Geometry: final body of the model. Coordinates: model frame, mm. A direction names the side the tool comes from. Give positions to 0.01 mm unless a question says otherwise; leave off trailing zeros. Order: outer loops, then holes, each group sorted by start corner. A loop starts at its lowest first (then second) coordinate and runs counter-clockwise, first axis right, second up. Notation, with made-up numbers: (0.25, 59) - (58.25, 59) arc R22 ccw to (58.25, 86) - close; hole circle Ø7 at (-33.75, 69). An arc over 180 degrees is marked (long way). Put each result on its own line as item: value. Start each with the question number.
1. Set-up query: faces 1 (the flat face through (4.1, 8, -9.6)), 2 (the flat face through (7.9, 8, -6.9)), 3 (the cylindrical face through (9.7, 2.96, -6.18)). Return all of +Z, -Z, +X, -X, +Y, -Y with unobstructed straight access to the full face (end or side cutting, diameter ignored); none if empty.
2. Section B-B on y = 9.5. Return the cut outline in (x, z).
3. Section C-C on z = 0. Return the cut outline in (x, y).
4. Section D-D on y = 2.5. Return the cut outline in (x, z), plus the area to 3 significant figures.
5. Section A-A on x = 0. Return the cut outline in (y, z), plus the area to 3 significant figures.
6. Ray query, line 1 along X through (y, z) = (2.75, 0); line 2 along Y through (x, z) = (-1.5, -2); line 3 along Y through (x, z) = (0, 4.75). Return the intervals inside material, ascending. Write a range as from..to.
7. First-contact query: P1, Ø5, axis at x = 0, z = 0, coming from the -Y side; P2, Ø8, axis at y = 2.5, z = -6, coming from the +X side; P3, Ø1.9, axis at y = 14.5, z = 0.5, coming from the +X side. Flat tips, straight axial feed; report the tip coordinate or a pass-through.
8. Mould query, pull axis Z, two halves, no side actions, for faces 4 (the cylindrical face through (-12.447, 2.465, 2.764)), 5 (the flat face through (0, 23.6, 0)), 6 (the flat face through (0, 11, 0)). Classes: pulls with the +Z half, pulls with the -Z half, needs draft (parallel to the pull), parting line crosses it, or undercut.
from build123d import *

# Parameters (mm, degrees)
SKETCH_1_R          = 14
EXTRUDE_1_DEPTH     = 10
SKETCH_2_R          = 11.5
CUT_EXTRUDE_1_DEPTH = 6
SKETCH_3_R          = 14
SKETCH_3_R_2        = 12.75
CUT_EXTRUDE_2_DEPTH = 5
CUT_EXTRUDE_START   = -4
CUT_EXTRUDE_3_DEPTH = 4
CHAMFER_1_SIZE      = 2
EXTRUDE_2_DEPTH     = 6.8
SKETCH_6_R          = 2.9
EXTRUDE_3_DEPTH     = 6.8
SKETCH_7_R          = 1.5
CUT_EXTRUDE_4_DEPTH = 5


with BuildPart() as part:
    # 草图1 → 凸台-拉伸1 (new body)
    with BuildSketch(Plane(origin=(0, 0, 0), x_dir=(1, 0, 0), z_dir=(0, 1, 0))):
        with Locations(Location((0, 0, 0), (0, 0, 270))):
            Circle(SKETCH_1_R)
    extrude(amount=EXTRUDE_1_DEPTH)

    # 草图2 → 切除-拉伸1 (cut)
    with BuildSketch(Plane.XZ):
        with Locations(Location((0, 0, 0), (0, 0, 270))):
            Circle(SKETCH_2_R)
    extrude(amount=-CUT_EXTRUDE_1_DEPTH, mode=Mode.SUBTRACT)

    # 草图3 → 切除-拉伸2 (cut)
    with BuildSketch(Plane.XZ):
        with Locations(Location((0, 0, 0), (0, 0, 270))):
            Circle(SKETCH_3_R)
        with Locations(Location((0, 0, 0), (0, 0, 270))):
            Circle(SKETCH_3_R_2, mode=Mode.SUBTRACT)
    extrude(amount=-CUT_EXTRUDE_2_DEPTH, mode=Mode.SUBTRACT)

    # 草图4 → 切除-拉伸3 (cut)
    with BuildSketch(Plane(origin=(0, 10, 0), x_dir=(1, 0, 0), z_dir=(0, 1, 0)).offset(CUT_EXTRUDE_START)):
        with BuildLine():
            Line((-5.46333165, 12.889996403), (-2.771638598, 6.39167453))
            ThreePointArc((-2.771638598, 6.39167453), (0, 4.539724827), (2.771638598, 6.39167453))
            Line((2.771638598, 6.39167453), (5.46333165, 12.889996403))
            ThreePointArc((5.46333165, 12.889996403), (0, 14), (-5.46333165, 12.889996403))
        make_face()
        with BuildLine():
            Line((-5.222360283, 4.611121001), (-10.570852749, 9.179165113))
            ThreePointArc((-10.570852749, 9.179165113), (-13.114723376, 4.899390856), (-14, 0))
            ThreePointArc((-14, 0), (-13.986838163, -0.6069252), (-13.9473774, -1.212709221))
            Line((-13.9473774, -1.212709221), (-6.935327141, -0.660848897))
            ThreePointArc((-6.935327141, -0.660848897), (-4.317534879, 1.402852121), (-5.222360283, 4.611121001))
        make_face()
        with BuildLine():
            Line((-5.999234754, -3.541845025), (-11.996477939, -7.216960375))
            ThreePointArc((-11.996477939, -7.216960375), (-8.228993532, -11.326237921), (-3.156621637, -13.63949192))
            Line((-3.156621637, -13.63949192), (-1.514629298, -6.800101609))
            ThreePointArc((-1.514629298, -6.800101609), (-2.668383303, -3.672714535), (-5.999234754, -3.541845025))
        make_face()
        with BuildLine():
            ThreePointArc((3.156621637, -13.63949192), (8.228993532, -11.326237921), (11.996477939, -7.216960375))
            Line((11.996477939, -7.216960375), (5.999234754, -3.541845025))
            ThreePointArc((5.999234754, -3.541845025), (2.668383303, -3.672714535), (1.514629298, -6.800101609))
            Line((1.514629298, -6.800101609), (3.156621637, -13.63949192))
        make_face()
        with BuildLine():
            ThreePointArc((14, 0), (13.114723376, 4.899390856), (10.570852749, 9.179165113))
            Line((10.570852749, 9.179165113), (5.222360283, 4.611121001))
            ThreePointArc((5.222360283, 4.611121001), (4.317534879, 1.402852121), (6.935327141, -0.660848897))
            Line((6.935327141, -0.660848897), (13.9473774, -1.212709221))
            ThreePointArc((13.9473774, -1.212709221), (13.986838163, -0.6069252), (14, 0))
        make_face()
    extrude(amount=CUT_EXTRUDE_3_DEPTH, mode=Mode.SUBTRACT)

    # 倒角1
    chamfer_1_edges = [part.edges().sort_by_distance(p)[0] for p in [
        (-8.228993532, 10, -11.326237921),
        (-13.314791228, 10, 4.326237921),
        (1.588570602, 10, 13.909580994),
        (13.314791228, 10, 4.326237921),
        (8.228993532, 10, -11.326237921),
    ]]
    chamfer(chamfer_1_edges, length=CHAMFER_1_SIZE)

    # 草图5 → 凸台-拉伸2 (add)
    with BuildSketch(Plane(origin=(0, 10, 0), x_dir=(1, 0, 0), z_dir=(0, 1, 0))):
        with BuildLine():
            Line((-3.45, 1.923538406), (-3.45, -1.923538406))
            ThreePointArc((-3.45, -1.923538406), (0, -3.95), (3.45, -1.923538406))
            Line((3.45, -1.923538406), (3.45, 1.923538406))
            ThreePointArc((3.45, 1.923538406), (0, 3.95), (-3.45, 1.923538406))
        make_face()
    extrude(amount=EXTRUDE_2_DEPTH)

    # 草图6 → 凸台-拉伸3 (add)
    with BuildSketch(Plane(origin=(0, 16.8, 0), x_dir=(1, 0, 0), z_dir=(0, 1, 0))):
        with Locations(Location((0, 0, 0), (0, 0, 270))):
            Circle(SKETCH_6_R)
    extrude(amount=EXTRUDE_3_DEPTH)

    # 草图7 → 切除-拉伸4 (cut)
    with BuildSketch(Plane.XZ.offset(-6)):
        with Locations(Location((0, 0, 0), (0, 0, 270))):
            Circle(SKETCH_7_R)
    extrude(amount=-CUT_EXTRUDE_4_DEPTH, mode=Mode.SUBTRACT)


solid = part.part
Resolved:
1. face 1: -Z, +Y
1. face 2: +X, +Y
1. face 3: -Y
2. outline: (-12.45, 1.1) - (-6.94, 0.66) arc R3 cw to (-5.22, -4.61) - (-9.43, -8.2) arc R12.5 ccw to (-4.89, -11.5) - (-2.77, -6.39) arc R3 cw to (2.77, -6.39) - (4.89, -11.5) arc R12.5 ccw to (9.43, -8.2) - (5.22, -4.61) arc R3 cw to (6.94, 0.66) - (12.45, 1.1) arc R12.5 ccw to (10.72, 6.43) - (6, 3.54) arc R3 cw to (1.51, 6.8) - (2.81, 12.18) arc R12.5 ccw to (-2.81, 12.18) - (-1.51, 6.8) arc R3 cw to (-6, 3.54) - (-10.72, 6.43) arc R12.5 ccw to start; hole circle Ø3 at (0, 0)
3. outline: (-14, 5) - (-12.75, 5) - (-12.75, 0) - (-11.5, 0) - (-11.5, 6) - (-14, 6) - close; (-5.28, 6) - (-1.5, 6) - (-1.5, 11) - (1.5, 11) - (1.5, 6) - (5.28, 6) - (5.28, 10) - (3.45, 10) - (3.45, 16.8) - (2.9, 16.8) - (2.9, 23.6) - (-2.9, 23.6) - (-2.9, 16.8) - (-3.45, 16.8) - (-3.45, 10) - (-5.28, 10) - close; (11.5, 0) - (12.75, 0) - (12.75, 5) - (14, 5) - (14, 6) - (11.5, 6) - close
4. outline: circle Ø25.5 at (0, 0); hole circle Ø23 at (0, 0)
4. area: 95.2 mm^2
5. outline: (0, -12.75) - (5, -12.75) - (5, -14) - (6, -14) - (6, -11.5) - (0, -11.5) - close; (0, 11.5) - (6, 11.5) - (6, 1.5) - (11, 1.5) - (11, -1.5) - (6, -1.5) - (6, -4.54) - (10, -4.54) - (10, -3.95) - (16.8, -3.95) - (16.8, -2.9) - (23.6, -2.9) - (23.6, 2.9) - (16.8, 2.9) - (16.8, 3.95) - (10, 3.95) - (10, 12) - (8, 14) - (5, 14) - (5, 12.75) - (0, 12.75) - close
5. area: 168 mm^2
6. line 1: -12.75..-11.5, 11.5..12.75
6. line 2: 6..23.6
6. line 3: 6..10
7. P1: y = 6
7. P2: x = 13.7
7. P3: x = 3.45
8. face 4: parting line crosses it
8. face 5: needs draft
8. face 6: undercut
